Model file for the job. Use its own axes, mm. Face numbers are marked on the shaded views. Coordinates: 2 decimals unless noted, no trailing zeros. Order: outer loops, then holes, each group sorted by start corner. A loop starts at its lowest first (then second) coordinate and runs counter-clockwise, first axis right, second up. Notation, with made-up numbers: M 26.25,-33 L 68.25,-33 A22 cw 68.25,-17 Z; hole C 35.5,59.25 d4. An arc over 180 degrees is marked long. Return JSON: item names as keys, results as strings.
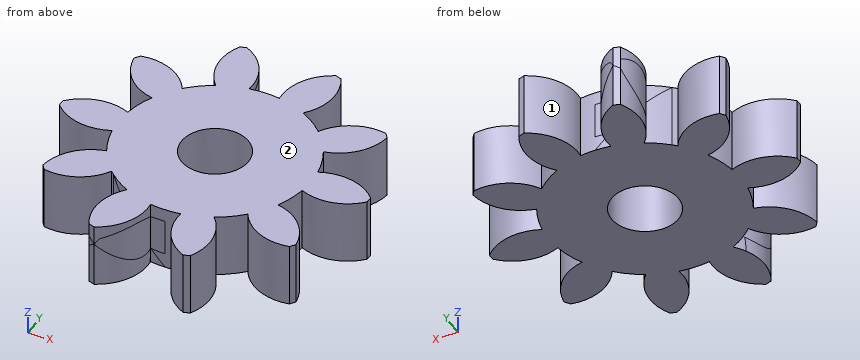
```python
from build123d import *

# Parameters (mm, degrees)
BASPROSKE_W                      = 5
BASPROSKE_H                      = 12
TOOTHCUT_DEPTH                   = 18.691806013
TEETHCUTS_COUNT                  = 10
TEETHCUTS_ANGLE                  = 324
BORSKE_R                         = 2.5
BORE_DEPTH                       = 50.0000508
S_LIDO_MOVER_COPIAR1_START       = -12
S_LIDO_MOVER_COPIAR1_OUTLINE_W   = 5
S_LIDO_MOVER_COPIAR1_OUTLINE_H   = 26
S_LIDO_MOVER_COPIAR1_DEPTH       = 12
S_LIDO_MOVER_COPIAR1_START_2     = 5
S_LIDO_MOVER_COPIAR1_2_OUTLINE_W = 5
S_LIDO_MOVER_COPIAR1_2_OUTLINE_H = 26
S_LIDO_MOVER_COPIAR1_2_DEPTH     = 7
S_LIDO_MOVER_COPIAR1_3_DEPTH     = 5
S_LIDO_MOVER_COPIAR1_4_OUTLINE_R = 2.5
S_LIDO_MOVER_COPIAR1_4_DEPTH     = 5
CROQUIS1_R                       = 2.6
CORTAR_EXTRUIR2_DEPTH            = 22.118885154


# Read off the part's stored shape, not the designer's step: Sólido-Mover/Copiar1
with BuildPart() as part:
    # BasProSke → Base-Revolve (revolve)
    with BuildSketch(Plane(origin=(0, 0, 0), x_dir=(1, 0, 0), z_dir=(0, 1, 0)), mode=Mode.PRIVATE) as base_revolve_sk:
        with Locations((2.5, 6)):
            Rectangle(BASPROSKE_W, BASPROSKE_H)
    revolve(base_revolve_sk.sketch.rotate(Axis((-10, 0, 0), (1, 0, 0)), 180), axis=Axis((-10, 0, 0), (1, 0, 0)))

    # TooCutSke → ToothCut (cut, through all)
    with BuildSketch(Plane(origin=(0, 0, 0), x_dir=(0, 0, -1), z_dir=(1, 0, 0))):
        with BuildLine():
            ThreePointArc((1.173662691, 7.406586048), (0, 7.499), (-1.173662691, 7.406586048))
            ThreePointArc((-1.173662691, 7.406586048), (-1.668191438, 9.834565786), (-3.497907776, 11.50542856))
            ThreePointArc((-3.497907776, 11.50542856), (0, 12.0254), (3.497907776, 11.50542856))
            ThreePointArc((3.497907776, 11.50542856), (1.668191438, 9.834565786), (1.173662691, 7.406586048))
        make_face()
    toothcut = extrude(amount=TOOTHCUT_DEPTH, mode=Mode.SUBTRACT)

    # TeethCuts: ToothCut ×10 about axis
    teethcuts_axis = Axis((-10, 0, 0), (1, 0, 0))
    for i in range(1, TEETHCUTS_COUNT):
        add(toothcut.rotate(teethcuts_axis, i * TEETHCUTS_ANGLE / (TEETHCUTS_COUNT - 1)), mode=Mode.SUBTRACT)

    # BorSke → Bore (cut, symmetric)
    with BuildSketch(Plane(origin=(0, 0, 0), x_dir=(0, 0, -1), z_dir=(1, 0, 0))):
        with Locations(Location((0, 0, 0), (0, 0, 180))):
            Circle(BORSKE_R)
    extrude(amount=BORE_DEPTH, both=True, mode=Mode.SUBTRACT)

    # Sólido-Mover/Copiar1 outline → Sólido-Mover/Copiar1 (cut)
    with BuildSketch(Plane.XY.offset(S_LIDO_MOVER_COPIAR1_START)):
        with Locations((2.5, 0)):
            Rectangle(S_LIDO_MOVER_COPIAR1_OUTLINE_W, S_LIDO_MOVER_COPIAR1_OUTLINE_H)
    extrude(amount=S_LIDO_MOVER_COPIAR1_DEPTH, mode=Mode.SUBTRACT)

    # S_lido-Mover_Copiar1 2 outline → S_lido-Mover_Copiar1 2 (cut)
    with BuildSketch(Plane.XY.offset(S_LIDO_MOVER_COPIAR1_START_2)):
        with Locations((2.5, 0)):
            Rectangle(S_LIDO_MOVER_COPIAR1_2_OUTLINE_W, S_LIDO_MOVER_COPIAR1_2_OUTLINE_H)
    extrude(amount=S_LIDO_MOVER_COPIAR1_2_DEPTH, mode=Mode.SUBTRACT)

    # S_lido-Mover_Copiar1 3 outline → S_lido-Mover_Copiar1 3 (cut)
    with BuildSketch(Plane.XY):
        with BuildLine():
            Line((0, 13), (0, 5.588828232))
            ThreePointArc((0, 5.588828232), (0.762620659, 6.187052394), (1.596031014, 6.681915604))
            ThreePointArc((1.596031014, 6.681915604), (0.571180494, 8.917819898), (1.0483384, 11.330682707))
            ThreePointArc((1.0483384, 11.330682707), (1.291796067, 11.412678196), (1.536953197, 11.489443278))
            ThreePointArc((1.536953197, 11.489443278), (3.341227227, 9.817862641), (3.826337309, 7.406586048))
            ThreePointArc((3.826337309, 7.406586048), (4.411352302, 7.475860812), (5, 7.499))
            Line((5, 7.499), (5, 13))
            Line((5, 13), (0, 13))
        make_face()
        with BuildLine():
            ThreePointArc((1.596031014, -6.681915604), (0.762620659, -6.187052394), (0, -5.588828232))
            Line((0, -5.588828232), (0, -13))
            Line((0, -13), (5, -13))
            Line((5, -13), (5, -7.499))
            ThreePointArc((5, -7.499), (4.411352302, -7.475860812), (3.826337309, -7.406586048))
            ThreePointArc((3.826337309, -7.406586048), (3.341227227, -9.817862641), (1.536953197, -11.489443278))
            ThreePointArc((1.536953197, -11.489443278), (1.291796067, -11.412678196), (1.0483384, -11.330682707))
            ThreePointArc((1.0483384, -11.330682707), (0.571180494, -8.917819898), (1.596031014, -6.681915604))
        make_face()
        with BuildLine():
            Line((5, -2.5), (5, 2.5))
            ThreePointArc((5, 2.5), (2.5, 0), (5, -2.5))
        make_face()
    extrude(amount=S_LIDO_MOVER_COPIAR1_3_DEPTH, mode=Mode.SUBTRACT)

    # S_lido-Mover_Copiar1 4 outline → S_lido-Mover_Copiar1 4 (add)
    with BuildSketch(Plane.XY):
        with BuildLine():
            ThreePointArc((-2.406763642, 1.172541409), (-4.849931218, 1.456299749), (-6.997250213, 0.256880001))
            ThreePointArc((-6.997250213, 0.256880001), (-7, 0), (-6.997250213, -0.256880001))
            ThreePointArc((-6.997250213, -0.256880001), (-4.849931218, -1.456299749), (-2.406763642, -1.172541409))
            ThreePointArc((-2.406763642, -1.172541409), (-2.131972816, -2.317318441), (-1.681400207, -3.404980509))
            ThreePointArc((-1.681400207, -3.404980509), (-3.824753264, -4.61147306), (-4.856969584, -6.843986457))
            ThreePointArc((-4.856969584, -6.843986457), (-4.708203933, -7.053423027), (-4.554989032, -7.259627029))
            ThreePointArc((-4.554989032, -7.259627029), (-2.112770233, -6.967815552), (-0.302995112, -5.302192362))
            ThreePointArc((-0.302995112, -5.302192362), (0.592198393, -6.066818441), (1.596031014, -6.681915604))
            ThreePointArc((1.596031014, -6.681915604), (0.571180494, -8.917819898), (1.0483384, -11.330682707))
            ThreePointArc((1.0483384, -11.330682707), (1.291796067, -11.412678196), (1.536953197, -11.489443278))
            ThreePointArc((1.536953197, -11.489443278), (3.341227227, -9.817862641), (3.826337309, -7.406586048))
            ThreePointArc((3.826337309, -7.406586048), (5, -7.499), (6.173662691, -7.406586048))
            ThreePointArc((6.173662691, -7.406586048), (6.658772773, -9.817862641), (8.463046803, -11.489443278))
            ThreePointArc((8.463046803, -11.489443278), (8.708203933, -11.412678196), (8.9516616, -11.330682707))
            ThreePointArc((8.9516616, -11.330682707), (9.428819506, -8.917819898), (8.403968986, -6.681915604))
            ThreePointArc((8.403968986, -6.681915604), (9.407801607, -6.066818441), (10.302995112, -5.302192362))
            ThreePointArc((10.302995112, -5.302192362), (12.112770233, -6.967815552), (14.554989032, -7.259627029))
            ThreePointArc((14.554989032, -7.259627029), (14.708203933, -7.053423027), (14.856969584, -6.843986457))
            ThreePointArc((14.856969584, -6.843986457), (13.824753264, -4.61147306), (11.681400207, -3.404980509))
            ThreePointArc((11.681400207, -3.404980509), (12.131972816, -2.317318441), (12.406763642, -1.172541409))
            ThreePointArc((12.406763642, -1.172541409), (14.849931218, -1.456299749), (16.997250213, -0.256880001))
            ThreePointArc((16.997250213, -0.256880001), (17, 0), (16.997250213, 0.256880001))
            ThreePointArc((16.997250213, 0.256880001), (14.849931218, 1.456299749), (12.406763642, 1.172541409))
            ThreePointArc((12.406763642, 1.172541409), (12.131972816, 2.317318441), (11.681400207, 3.404980509))
            ThreePointArc((11.681400207, 3.404980509), (13.824753264, 4.61147306), (14.856969584, 6.843986457))
            ThreePointArc((14.856969584, 6.843986457), (14.708203933, 7.053423027), (14.554989032, 7.259627029))
            ThreePointArc((14.554989032, 7.259627029), (12.112770233, 6.967815552), (10.302995112, 5.302192362))
            ThreePointArc((10.302995112, 5.302192362), (9.407801607, 6.066818441), (8.403968986, 6.681915604))
            ThreePointArc((8.403968986, 6.681915604), (9.428819506, 8.917819898), (8.9516616, 11.330682707))
            ThreePointArc((8.9516616, 11.330682707), (8.708203933, 11.412678196), (8.463046803, 11.489443278))
            ThreePointArc((8.463046803, 11.489443278), (6.658772773, 9.817862641), (6.173662691, 7.406586048))
            ThreePointArc((6.173662691, 7.406586048), (5, 7.499), (3.826337309, 7.406586048))
            ThreePointArc((3.826337309, 7.406586048), (3.341227227, 9.817862641), (1.536953197, 11.489443278))
            ThreePointArc((1.536953197, 11.489443278), (1.291796067, 11.412678196), (1.0483384, 11.330682707))
            ThreePointArc((1.0483384, 11.330682707), (0.571180494, 8.917819898), (1.596031014, 6.681915604))
            ThreePointArc((1.596031014, 6.681915604), (0.592198393, 6.066818441), (-0.302995112, 5.302192362))
            ThreePointArc((-0.302995112, 5.302192362), (-2.112770233, 6.967815552), (-4.554989032, 7.259627029))
            ThreePointArc((-4.554989032, 7.259627029), (-4.708203933, 7.053423027), (-4.856969584, 6.843986457))
            ThreePointArc((-4.856969584, 6.843986457), (-3.824753264, 4.61147306), (-1.681400207, 3.404980509))
            ThreePointArc((-1.681400207, 3.404980509), (-2.131972816, 2.317318441), (-2.406763642, 1.172541409))
        make_face()
        with Locations((5, 0)):
            Circle(S_LIDO_MOVER_COPIAR1_4_OUTLINE_R, mode=Mode.SUBTRACT)
    extrude(amount=S_LIDO_MOVER_COPIAR1_4_DEPTH)

    # Croquis1 → Cortar-Extruir2 (cut, through all)
    with BuildSketch(Plane.XY.offset(5)):
        with Locations((5, 0)):
            Circle(CROQUIS1_R)
    extrude(amount=-CORTAR_EXTRUIR2_DEPTH, mode=Mode.SUBTRACT)


solid = part.part
```
Item 1: Saw through at C-C (x = 14). Write the cut outline in (y, z), and give its area (3 significant figures).
Check result:
{"outline": "M -7.33,0 L -4.81,0 L -4.81,5 L -7.33,5 Z; M -1.53,0 L 1.53,0 L 1.53,5 L -1.53,5 Z; M 4.81,0 L 7.33,0 L 7.33,5 L 4.81,5 Z", "area": "40.5 mm2"}
Item 2: Saw through at B-B (x = 4.25). Write the cut outline in (y, z).
Check result:
{"outline": "M -7.46,0 L -2.49,0 L -2.49,5 L -7.46,5 Z; M 2.49,0 L 7.46,0 L 7.46,5 L 2.49,5 Z"}
Item 3: Pull direction X, two halves, no side cores. Call the marked faces 1 and 2: +X half, -X half, draft (parallel to the pull), parting line (faces both ways), or undercut.
Check result:
{"face 1": "undercut", "face 2": "draft"}
Item 4: Wall check: line 1 (Y direction, x = 5, z = 2.3); line 2 (Y direction, x = 12.75, z = 1.3); line 3 (Y direction, x = 4.25, z = 3.95). Give the ranges that are in metal, low to high.
Check result:
{"line 1": "y = -7.5 to -2.6, 2.6 to 7.5", "line 2": "y = -7.2 to -3.79, -1.31 to 1.31, 3.79 to 7.2", "line 3": "y = -7.46 to -2.49, 2.49 to 7.46"}
Item 5: Saw through at A-A (y = 2). Write the cut outline in (x, z).
Check result:
{"outline": "M -2.23,0 L 3.34,0 L 3.34,5 L -2.23,5 Z; M 6.66,0 L 12.23,0 L 12.23,5 L 6.66,5 Z"}
Item 6: Drop flat-ended pins along their axis: pin 1 Ø2 at (y, z) = (-7.5, 1.5) entering from -X; pin 2 Ø3 at (x, z) = (5, 3) entering from +Y; pin 3 Ø4.5 at (x, y) = (5, 0) entering from -Z; pin 4 Ø1.5 at (x, z) = (0.5, 1) entering from -Y. Give the stop position or say it passes through.
Check result:
{"pin 1": "stops at x = -4.86", "pin 2": "stops at y = 9.5", "pin 3": "passes through", "pin 4": "stops at y = -11.4"}
Item 7: Saw through at D-D (y = -5). Write the cut outline in (x, z).
Check result:
{"outline": "M -4.14,0 L 14.14,0 L 14.14,5 L -4.14,5 Z"}
